```python
from build123d import *

# Parameters (mm, degrees)
ESBO_O2_R                = 3.75
RESSALTO_EXTRUS_O6_DEPTH = 2.24
ESBO_O2_6_R              = 12.055555556
RESSALTO_EXTRUS_O7_DEPTH = 3
FILETE3_R                = 0.1


with BuildPart() as part:
    # Esboço2 → Ressalto-extrusão6 (new body)
    with BuildSketch(Plane.XY):
        with BuildLine():
            ThreePointArc((-1.286579516, 7.388823529), (-6.144565705, 4.3005014), (-7.382691193, -1.321314024))
            ThreePointArc((-7.382691193, -1.321314024), (-5.290815774, -5.31575662), (-1.286579516, -7.388823529))
            ThreePointArc((-1.286579516, -7.388823529), (0, -6.8), (1.286579516, -7.388823529))
            ThreePointArc((1.286579516, -7.388823529), (6.144565705, -4.3005014), (7.382691193, 1.321314024))
            ThreePointArc((7.382691193, 1.321314024), (5.290815774, 5.31575662), (1.286579516, 7.388823529))
            ThreePointArc((1.286579516, 7.388823529), (0, 6.8), (-1.286579516, 7.388823529))
        make_face()
        Circle(ESBO_O2_R, mode=Mode.SUBTRACT)
    extrude(amount=RESSALTO_EXTRUS_O6_DEPTH)

    # Esboço2<6> → Ressalto-extrusão7 (add)
    with BuildSketch(Plane.XY):
        Circle(ESBO_O2_6_R)
        with BuildLine():
            ThreePointArc((-1.286579516, -7.388823529), (-5.290815774, -5.31575662), (-7.382691193, -1.321314024))
            ThreePointArc((-7.382691193, -1.321314024), (-6.144565705, 4.3005014), (-1.286579516, 7.388823529))
            ThreePointArc((-1.286579516, 7.388823529), (-0.592796265, 10.09329614), (1.7, 8.5))
            ThreePointArc((1.7, 8.5), (1.59329614, 7.907203735), (1.286579516, 7.388823529))
            ThreePointArc((1.286579516, 7.388823529), (5.290815774, 5.31575662), (7.382691193, 1.321314024))
            ThreePointArc((7.382691193, 1.321314024), (6.144565705, -4.3005014), (1.286579516, -7.388823529))
            ThreePointArc((1.286579516, -7.388823529), (1.59329614, -7.907203735), (1.7, -8.5))
            ThreePointArc((1.7, -8.5), (-0.592796265, -10.09329614), (-1.286579516, -7.388823529))
        make_face(mode=Mode.SUBTRACT)
    extrude(amount=RESSALTO_EXTRUS_O7_DEPTH)

    # Filete3
    filete3_edges = [part.edges().sort_by_distance(p)[0] for p in [
        (7.5, 0, 3),
        (-7.5, 0, 3),
        (-0.592796265, 10.09329614, 3),
        (0, -10.2, 3),
    ]]
    fillet(filete3_edges, radius=FILETE3_R)


solid = part.part
```
Check sheet for the modelled part. Datum: model origin and axes. Units: mm. Round coordinates to 2 decimals unless told otherwise and drop trailing zeros. Order: outer loops, then holes, each group sorted by start corner. A loop starts at its lowest first (then second) coordinate and runs counter-clockwise, first axis right, second up. Notation, with made-up numbers: (60.25, 60) -> (103.25, 60) arc R18 cw to (103.25, 67) -> close; hole circle Ø11 at (-1.75, -1). An arc over 180 degrees is marked (long way). One line per item, written item: value. Start each with the question number.
Q1. Thickness scan on line 1 (X direction, y = 2, z = 2.85); line 2 (X direction, y = -1.5, z = 1.9); line 3 (Y direction, x = 4.5, z = 1.85). Record the ranges inside material, lowest first.
Q2. Mould release check, pull along X, two halves, no side actions. Record for faces 1 (the face through (6.481, 10.165, 1.479)), 2 (the face through (3, 3, 0)), 3 (the face through (3, -3, 2.24)): pulls with the +X half, pulls with the -X half, needs draft (parallel to the pull), parting line crosses it, or undercut.
Q3. Cross-section at B-B (x = 0). Give the number of separate pieces and of enclosed holes in the cut face, and give its area (3 significant figures).
Q4. Cross-section at A-A (z = 1.45). Record the boundary of the cut face in (x, y).
Q5. Cross-section at C-C (x = 9.5). Record the boundary of the cut face in (y, z).
Q6. Gauge pin test, flat ends, axial feed: pin 1 Ø1 at (x, z) = (5, 2.5) entering from +Y; pin 2 Ø7 at (x, y) = (0, 0) entering from -Z; pin 3 Ø4.5 at (x, y) = (0, 3.5) entering from +Z; pin 4 Ø2 at (x, y) = (4.5, 0) entering from -Z. Record the tip position at first contact, or that the pin passes through.
Completed:
1. line 1: x = -11.89 to -7.23, 7.23 to 11.89
1. line 2: x = -11.96 to -3.44, 3.44 to 11.96
1. line 3: y = -11.18 to 11.18
2. face 1: parting line crosses it
2. face 2: needs draft
2. face 3: undercut
3. separate pieces: 4
3. enclosed holes: 0
3. area: 24.8 mm²
4. outline: circle Ø24.11 at (0, 0); hole circle Ø7.5 at (0, 0); hole circle Ø3.4 at (0, -8.5); hole circle Ø3.4 at (0, 8.5)
5. outline: (-7.42, 0) -> (7.42, 0) -> (7.42, 3) -> (-7.42, 3) -> close
6. pin 1: stops at y = 11.18
6. pin 2: passes through
6. pin 3: stops at z = 2.24
6. pin 4: stops at z = 0
